Autodesk Inventor part; units mm, degrees
ref_plane "YZ Plane" through (0, 0, 0) normal (1, 0, 0) x (0, 1, 0)
ref_plane "XZ Plane" through (0, 0, 0) normal (0, 1, 0) x (-1, 0, 0)
ref_plane "XY Plane" through (0, 0, 0) normal (0, 0, 1) x (1, 0, 0)
ref_plane "Work Plane1" through (0, 0, 0) normal (0, 0, 1) x (1, 0, 0)
sketch "Sketch1" plane through (0, 0, 0) normal (0, 0, 1) x (1, 0, 0)
  circle A0 centre (6.5, 20.75) radius 1
  circle A1 centre (6.5, 4.75) radius 1
  circle A2 centre (22.5, 20.75) radius 1
  circle A3 centre (22.5, 4.75) radius 1
  line L0 (-13, -14.75) -> (43.896, -14.75)
  line L1 (43.896, -14.75) -> (43.896, 40.25)
  line L2 (43.896, 40.25) -> (-13, 40.25)
  line L3 (-13, 40.25) -> (-13, -14.75)
  circle A4 centre (22.5, 12.75) radius 1
  circle A5 centre (14.5, 20.75) radius 1
  circle A6 centre (14.5, 4.75) radius 1
  circle A7 centre (6.5, 12.75) radius 1
  point P0 (0, 0)
  point P1 (14.5, 12.75)
  dimension "d1" = 55
  dimension "d100" = 29.396
  dimension "d101" = 27.5
  dimension "d104" = 2
  dimension "d105" = 2
  dimension "d106" = 2
  dimension "d107" = 2
extrude "Extrusion3" add sketch "Sketch1" along normal blind 3
sketch "Sketch4" plane through (0, 0, 3) normal (0, 0, 1) x (1, 0, 0)
  line L0 (42, 40.25) -> (-13, 40.25) construction
  line L1 (14.5, 40.25) -> (14.5, 12.75) construction
  line L2 (-13, -14.75) -> (42, -14.75) construction
  line L3 (-13, 40.25) -> (-13, -14.75) construction
  line L4 (-13, 12.75) -> (14.5, 12.75) construction
  circle A0 centre (14.5, 30.75) radius 3.895
  circle A1 centre (1.7721, 25.4779) radius 3.895
  circle A2 centre (-3.5, 12.75) radius 3.895
  circle A3 centre (1.7721, 0.0221) radius 3.895
  circle A4 centre (14.5, -5.25) radius 3.895
  circle A5 centre (27.2279, 0.0221) radius 3.895
  circle A6 centre (32.5, 12.75) radius 3.895
  circle A7 centre (27.2279, 25.4779) radius 3.895
  arc A8 (4.6716, 35.75) -> (4.6716, 37.75) centre (7.5, 36.75) ccw
  line L5 (42, 40.25) -> (-13, 40.25)
  line L6 (7.5, 36.75) -> (-13, 36.75) construction
  line L7 (4.6716, 37.75) -> (-7.3284, 37.75)
  line L8 (4.6716, 35.75) -> (-7.3284, 35.75)
  line L9 (-7.3284, 37.75) -> (-7.3284, 40.25)
  line L10 (10.9716, 40.25) -> (-7.3284, 40.25)
  line L11 (-7.3284, 35.75) -> (-7.3284, 33.25)
  line L12 (-7.3284, 33.25) -> (10.9716, 33.25)
  line L13 (10.9716, 40.25) -> (10.9716, 33.25)
  arc A9 (24.3284, 37.75) -> (24.3284, 35.75) centre (21.5, 36.75) ccw
  line L14 (24.3284, 37.75) -> (36.3284, 37.75)
  line L15 (24.3284, 35.75) -> (36.3284, 35.75)
  line L16 (36.3284, 37.75) -> (36.3284, 40.25)
  line L17 (18.0284, 40.25) -> (36.3284, 40.25)
  line L18 (36.3284, 35.75) -> (36.3284, 33.25)
  line L19 (36.3284, 33.25) -> (18.0284, 33.25)
  line L20 (18.0284, 40.25) -> (18.0284, 33.25)
  arc A10 (-6.6716, -10.25) -> (-6.6716, -12.25) centre (-9.5, -11.25) ccw
  line L21 (-9.5, -11.25) -> (8.4531, -11.25) construction
  line L22 (-6.6716, -10.25) -> (5.3284, -10.25)
  line L23 (-6.6716, -12.25) -> (5.3284, -12.25)
  line L24 (5.3284, -12.25) -> (5.3284, -14.75)
  line L25 (5.3284, -10.25) -> (5.3284, -7.75)
  line L26 (5.3284, -7.75) -> (-13, -7.75)
  line L27 (-13, -14.75) -> (-13, -7.75)
  line L28 (-13, -14.75) -> (5.3284, -14.75)
  circle A11 centre (14.5, 12.75) radius 5
  point P0 (0, 0)
  dimension "d24" = 7.79
  dimension "d25" = 18
  dimension "d28" = 360
  dimension "d63" = 6
  dimension "d64" = 7
  dimension "d65" = 12
  dimension "d66" = 18.3
  dimension "d67" = 2.5
  dimension "d68" = 3.5
  dimension "d71" = 1
  dimension "d74" = 6
  dimension "d75" = 3.5
  dimension "d76" = 3.5
  dimension "d77" = 12
  dimension "d78" = 1
  dimension "d79" = 2.5
  dimension "d102" = 10
extrude "Extrusion2" cut sketch "Sketch4" against normal through all
hole "Hole4" at (7.5, 36.75, 3) at (21.5, 36.75, 3) at (-9.5, -11.25, 3) direction (0, 0, -1) diameter 2 end through all
fillet "Fillet3" radius 2 14 edges at (-7.3284, 35.75, 1.5) (-7.3284, 37.75, 1.5) (4.6716, 37.75, 1.5) (4.6716, 35.75, 1.5) (10.9716, 33.25, 1.5) (24.3284, 37.75, 1.5) (24.3284, 35.75, 1.5) (36.3284, 37.75, 1.5) (36.3284, 35.75, 1.5) (18.0284, 33.25, 1.5) (5.3284, -10.25, 1.5) (5.3284, -12.25, 1.5) (-6.6716, -10.25, 1.5) (-6.6716, -12.25, 1.5)
sketch "Sketch6" plane through (0, 0, 3) normal (0, 0, 1) x (1, 0, 0)
  line L0 (43.896, 40.25) -> (36.3284, 40.25)
  line L1 (43.896, 40.25) -> (40.796, 40.25)
  line L2 (40.796, 40.25) -> (40.796, 20.2)
  line L3 (40.796, 20.2) -> (43.896, 20.2)
  line L4 (43.896, 20.2) -> (43.896, 40.25)
  line L5 (43.896, -14.75) -> (43.896, 40.25) construction
  line L6 (43.896, 12.75) -> (-13, 12.75) construction
  line L7 (-13, 40.25) -> (-13, -7.75) construction
  line L8 (43.896, -14.75) -> (40.796, -14.75)
  line L9 (40.796, -14.75) -> (40.796, 5.3)
  line L10 (40.796, 5.3) -> (43.896, 5.3)
  line L11 (43.896, 5.3) -> (43.896, -14.75)
  point P0 (0, 0)
  dimension "d96" = 3.1
  dimension "d97" = 20.05
extrude "Extrusion4" cut sketch "Sketch6" against normal through all
fillet "Fillet4" radius 3 1 edges at (-13, 40.25, 1.5)
equation "\"d38\" = d24"
properties part number "SideB"
Check sheet for the modelled part. Datum: model origin and axes. Units: mm. A direction names the side the tool comes from. Give positions to 0.01 mm unless a question says otherwise; leave off trailing zeros. Loops run counter-clockwise (first coordinate to the right, second up) from the corner with the lowest first, then second, coordinate; pieces in that order, holes last. Notation, with made-up numbers: M 34,31.5 L 48,31.5 A24 ccw 48,64.5 Z; hole C 45.5,-31 d3. An arc over 180 degrees is marked long. Answer as a JSON object with one key per item and string values. Group by question number.
Q1. Cross-section at B-B on x = 32.5. Record the cut outline in (y, z) (3 decimals), then the cut area to 3 significant figures.
Q2. Cross-section at A-A on y = 12.75. Record the cut outline in (x, z) (3 decimals).
Q3. Cross-section at C-C on y = -11.25. Record the cut outline in (x, z).
Q4. Cross-section at D-D on z = 1.4. Give the number of separate pieces and of enclosed holes in the cut face, then the cut area to 3 significant figures.
Q5. Material ranges on line 1 along X through (y, z) = (36.75, 0.85); line 2 along Y through (x, z) = (2, 1); line 3 along Y through (x, z) = (-9.5, 1.45), recorded low to high. Write a range as [from, to].
Q6. Access from +Z, -Z, +X, -X, +Y, -Y to the whole of each face (thin tool, end or side, straight path). Record for faces 5 (the flat face through (40.796, 30, 2)), 6 (the flat face through (43.896, 13, 1)), 7 (the flat face through (1, 33.25, 2)).
Q7. Release check for a two-part mould opening along Y. For faces 1 (the cylindrical face through (23.337, 0.193, 1.521)), 2 (the flat face through (40.796, -5, 2)), 3 (the cylindrical face through (35.758, 38.351, 1.479)), 4 (the cylindrical face through (13.656, 26.948, 1.521)) record: released by +Y, released by -Y, zero draft, split by the parting line, or undercut.
Q8. Go/stop test with flat-tipped pins: P1, Ø1, axis at x = 26, z = 1, coming from the +Y side; P2, Ø0.6, axis at y = 40, z = 2, coming from the -X side. Record where each tip stops, or that it passes through.
Evaluation:
{
 "1": {"outline": "M -14.75,0 L 8.855,0 L 8.855,3 L -14.75,3 Z; M 16.645,0 L 33.25,0 L 33.25,3 L 16.645,3 Z; M 35.75,0 L 37.75,0 L 37.75,3 L 35.75,3 Z", "area": "127 mm2"},
 "2": {"outline": "M -13,0 L -7.395,0 L -7.395,3 L -13,3 Z; M 0.395,0 L 5.5,0 L 5.5,3 L 0.395,3 Z; M 7.5,0 L 9.5,0 L 9.5,3 L 7.5,3 Z; M 19.5,0 L 21.5,0 L 21.5,3 L 19.5,3 Z; M 23.5,0 L 28.605,0 L 28.605,3 L 23.5,3 Z; M 36.395,0 L 43.896,0 L 43.896,3 L 36.395,3 Z"},
 "3": {"outline": "M -12.5,0 L -10.5,0 L -10.5,3 L -12.5,3 Z; M -8.5,0 L 40.8,0 L 40.8,3 L -8.5,3 Z"},
 "4": {"separate pieces": "1", "enclosed holes": "20", "area": "2,290 mm2"},
 "5": {"line 1": "x = [-13, 6.5], [8.5, 10.5], [10.97, 18.03], [18.5, 20.5], [22.5, 40.8]", "line 2": "y = [-12.25, -10.25], [-7.75, -3.87], [3.91, 21.59], [29.37, 33.25], [35.75, 37.75]", "line 3": "y = [-14.25, -12.25], [-10.25, -8.25], [-7.75, 40.25]"},
 "6": {"face 5": "+Z, -Z, +X, +Y", "face 6": "+Z, -Z, +X, +Y, -Y", "face 7": "+Z, -Z"},
 "7": {"face 1": "undercut", "face 2": "zero draft", "face 3": "released by +Y", "face 4": "undercut"},
 "8": {"P1": "stops at y = 37.75", "P2": "stops at x = -11.73"}
}
